Geometry: see drawing. Coordinates: mm, zero at the bounding-box minimum. A direction names the side the tool comes from. Give positions to 0.01 mm unless a question says otherwise; leave off trailing zeros. Loops run counter-clockwise (first coordinate to the right, second up) from the corner with the lowest first, then second, coordinate; pieces in that order, holes last. Notation, with made-up numbers: M 80,41 L 98,41 A32 ccw 98,67 Z; hole C 43,84 d8. An arc over 180 degrees is marked long. Put each result on its own line as item: value.
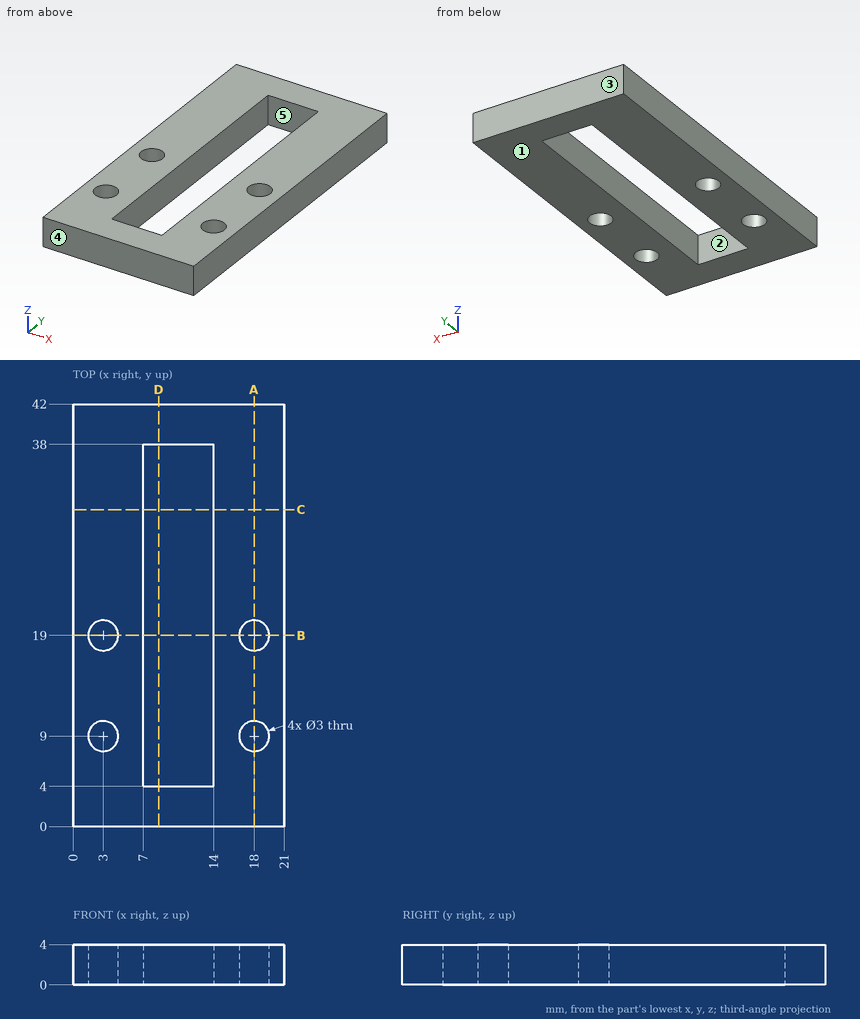
1. Section query D-D (x = 8.5). Output: boundary loops of the cut face in (y, z).
Found:
outline: M 0,0 L 4,0 L 4,4 L 0,4 Z; M 38,0 L 42,0 L 42,4 L 38,4 Z
2. Draft query along Y for the marked faces 3, 4 and 5. Return one class per face: pulls with the +Y half, pulls with the -Y half, needs draft (parallel to the pull), parting line crosses it, or undercut.
Found:
face 3: pulls with the +Y half
face 4: pulls with the -Y half
face 5: undercut
3. Section query A-A (x = 18). Output: boundary loops of the cut face in (y, z).
Found:
outline: M 0,0 L 7.5,0 L 7.5,4 L 0,4 Z; M 10.5,0 L 17.5,0 L 17.5,4 L 10.5,4 Z; M 20.5,0 L 42,0 L 42,4 L 20.5,4 Z
4. Material intervals for line 1 (Y direction, x = 18, z = 2.15); line 2 (X direction, y = 36.5, z = 2.85); line 3 (Y direction, x = 9, z = 1.65), sorted ascending. Write a range as from..to.
Found:
line 1: 0..7.5, 10.5..17.5, 20.5..42
line 2: 0..7, 14..21
line 3: 0..4, 38..42
5. Access query for the marked faces 1 and 2. Directions: +Z, -Z, +X, -X, +Y, -Y. A direction counts if a zero-diameter tool reaches every point of the face in a straight line with its end or side. Return the directions, or none.
Found:
face 1: -Z, +X, -X, +Y, -Y
face 2: +Z, -Z
6. Section query B-B (y = 19). Output: boundary loops of the cut face in (x, z), plus the area to 3 significant figures.
Found:
outline: M 0,0 L 1.5,0 L 1.5,4 L 0,4 Z; M 4.5,0 L 7,0 L 7,4 L 4.5,4 Z; M 14,0 L 16.5,0 L 16.5,4 L 14,4 Z; M 19.5,0 L 21,0 L 21,4 L 19.5,4 Z
area: 32.0 mm^2
7. Section query C-C (y = 31.5). Output: boundary loops of the cut face in (x, z).
Found:
outline: M 0,0 L 7,0 L 7,4 L 0,4 Z; M 14,0 L 21,0 L 21,4 L 14,4 Z
